Check sheet for the modelled part. Datum: model origin and axes. Units: mm. Round coordinates to 2 decimals unless told otherwise and drop trailing zeros. Write each loop counter-clockwise with the first axis right and the second up, starting at its lowest first coordinate (ties: lowest second). Pieces come first, ordered by that corner, then holes. Notation, with made-up numbers: (-3, -16) -> (26, -16) arc R23 ccw to (26, 20) -> close; hole circle Ø7 at (31, -8). An arc over 180 degrees is marked (long way). Answer as a JSON object with one key per item and string values. Group by question number.
```python
from build123d import *

# Parameters (mm, degrees)
BOSS_EXTRUDE2_DEPTH = 3
SKETCH3_R           = 1.5
SKETCH3_R_2         = 7.46
CUT_EXTRUDE1_DEPTH  = 3


with BuildPart() as part:
    # Sketch2 → Boss-Extrude2 (new body)
    with BuildSketch(Plane.XY):
        with BuildLine():
            Line((116.251704746, 156.353577499), (112.006054704, 154.834164358))
            Line((112.006054704, 154.834164358), (102.590821765, 141.464685362))
            Line((102.590821765, 141.464685362), (102.590821765, 86.213632981))
            Line((102.590821765, 86.213632981), (111.385068158, 71.453251655))
            Line((111.385068158, 71.453251655), (116.251704746, 68.818910417))
            ThreePointArc((116.251704746, 68.818910417), (123.784731531, 67.289899242), (131.464672299, 66.969153974))
            ThreePointArc((131.464672299, 66.969153974), (139.129294477, 67.550475385), (146.606062492, 69.334377784))
            Line((146.606062492, 69.334377784), (151.380447861, 72.132439574))
            Line((151.380447861, 72.132439574), (159.66845659, 87.18290594))
            Line((159.66845659, 87.18290594), (157.79248846, 142.402101269))
            Line((157.79248846, 142.402101269), (147.928743251, 155.444191223))
            Line((147.928743251, 155.444191223), (143.63395176, 156.818573493))
            ThreePointArc((143.63395176, 156.818573493), (136.819761385, 157.949780649), (129.915894372, 158.172132571))
            ThreePointArc((129.915894372, 158.172132571), (123.023557673, 157.715498216), (116.251704746, 156.353577499))
        make_face()
    extrude(amount=BOSS_EXTRUDE2_DEPTH)

    # Sketch3 → Cut-Extrude1 (cut)
    with BuildSketch(Plane.XY.offset(3)):
        with Locations((106.270821765, 132.294685362)):
            Circle(SKETCH3_R)
        with Locations((106.270821765, 92.943632981)):
            Circle(SKETCH3_R)
        with Locations((154.065868873, 132.294685362)):
            Circle(SKETCH3_R)
        with Locations((154.065868873, 92.943632981)):
            Circle(SKETCH3_R)
        with Locations((131.66355574, 112.585551326)):
            Circle(SKETCH3_R_2)
    extrude(amount=-CUT_EXTRUDE1_DEPTH, mode=Mode.SUBTRACT)


solid = part.part
```
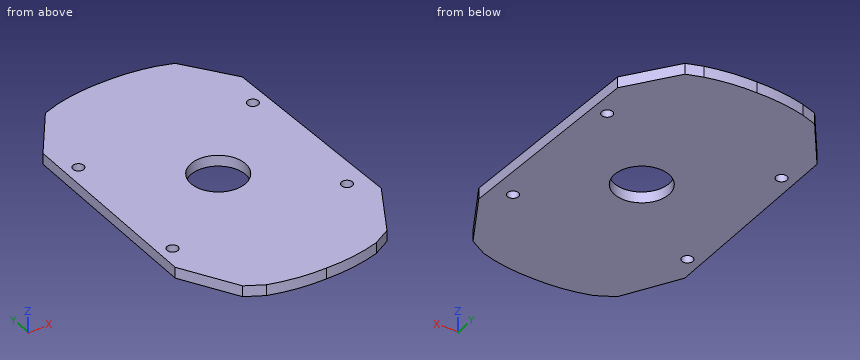
(1) Go/stop test with flat-tipped pins: pin 1 Ø1.5 at (x, z) = (110.5, 1) entering from -Y; pin 2 Ø1.8 at (x, y) = (154.07, 92.94) entering from +Z; pin 3 Ø1.5 at (y, z) = (116.5, 0.5) entering from +X. Record where each tip stops, or that it passes through.
(2) Section check D-D on y = 128.5. Record the cut outline in (x, z).
(3) Section check A-A on y = 109. Record the cut outline in (x, z).
(4) Section check C-C on x = 128. Record the cut outline in (y, z).
(5) Scan lines: line 1 along X through (y, z) = (133, 1.85); line 2 along Y through (x, z) = (154.5, 0.3); line 3 along X through (y, z) = (130.5, 1.7). Record each from-to range of solid material in increasing order.
(6) Section check B-B on z = 1.7. Record the cut outline in (x, y).
Data:
{
 "1": {"pin 1": "stops at y = 71.68", "pin 2": "passes through", "pin 3": "stops at x = 158.7"},
 "2": {"outline": "(102.59, 0) -> (158.26, 0) -> (158.26, 3) -> (102.59, 3) -> close"},
 "3": {"outline": "(102.59, 0) -> (125.12, 0) -> (125.12, 3) -> (102.59, 3) -> close; (138.21, 0) -> (158.93, 0) -> (158.93, 3) -> (138.21, 3) -> close"},
 "4": {"outline": "(66.96, 0) -> (106.09, 0) -> (106.09, 3) -> (66.96, 3) -> close; (119.08, 0) -> (158.14, 0) -> (158.14, 3) -> (119.08, 3) -> close"},
 "5": {"line 1": "x = 102.59 to 104.95, 107.59 to 152.74, 155.39 to 158.11", "line 2": "y = 77.8 to 91.51, 94.38 to 130.86, 133.73 to 146.76", "line 3": "x = 102.59 to 158.2"},
 "6": {"outline": "(102.59, 86.21) -> (111.39, 71.45) -> (116.25, 68.82) arc R48.54 ccw to (131.46, 66.97) arc R48.54 ccw to (146.61, 69.33) -> (151.38, 72.13) -> (159.67, 87.18) -> (157.79, 142.4) -> (147.93, 155.44) -> (143.63, 156.82) arc R52.24 ccw to (129.92, 158.17) arc R52.24 ccw to (116.25, 156.35) -> (112.01, 154.83) -> (102.59, 141.46) -> close; hole circle Ø3 at (106.27, 92.94); hole circle Ø3 at (106.27, 132.29); hole circle Ø14.92 at (131.66, 112.59); hole circle Ø3 at (154.07, 92.94); hole circle Ø3 at (154.07, 132.29)"}
}
